from build123d import *

# Parameters (mm, degrees)
F1_DEPTH = 500
F2_W     = 221.745663
F2_H     = 538.323703
F2_R     = 1.9
F3_DEPTH = 50
F4_W     = 4.4
F4_H     = 51
F4_W_2   = 12.8
F4_R     = 1.9
F5_DEPTH = 1


with BuildPart() as f1:
    # F0 (on Front) → F1 (new body)
    with BuildSketch(Plane.XZ):
        with BuildLine():
            Line((-20, 3), (-20, 42))
            Line((-20, 42), (-23, 42))
            Line((-23, 42), (-23, 3))
            ThreePointArc((-23, 3), (-21.242641, -1.242641), (-17, -3))
            Line((-17, -3), (127, -3))
            Line((127, -3), (127, 0))
            Line((127, 0), (-17, 0))
            ThreePointArc((-17, 0), (-19.12132, 0.87868), (-20, 3))
        make_face()
    extrude(amount=-F1_DEPTH)

    # F2 (on Top) → F3 (cut, symmetric)
    with BuildSketch(Plane.XY):
        with Locations((54.499505, 256.060087)):
            Rectangle(F2_W, F2_H)
        with BuildLine():
            Line((126.619398, 279.652744), (33.186834, 54.086583))
            ThreePointArc((33.186834, 54.086583), (31.345288, 51.842652), (28.567437, 51))
            Line((28.567437, 51), (-3.3, 51))
            ThreePointArc((-3.3, 51), (-5.421321, 50.12132), (-6.3, 48))
            Line((-6.3, 48), (-6.3, 0))
            Line((-6.3, 0), (-16, 0))
            Line((-16, 0), (-16, 16))
            ThreePointArc((-16, 16), (-16.87868, 18.12132), (-19, 19))
            Line((-19, 19), (-23, 19))
            Line((-23, 19), (-23, 397))
            ThreePointArc((-23, 397), (-20.832031, 401.120631), (-16.20816, 401.667902))
            Line((-16.20816, 401.667902), (123.79184, 347.926937))
            ThreePointArc((123.79184, 347.926937), (126.120631, 346.091066), (127, 343.259035))
            Line((127, 343.259035), (127, 281.566161))
            ThreePointArc((127, 281.566161), (126.903926, 280.59071), (126.619398, 279.652744))
        make_face(mode=Mode.SUBTRACT)
        Polygon((467.411696, 344.689719), (455.614504, 344.432303), (456.010659, 326.276753), (456.727063, 293.44444), (469.524017, 293.72367), (468.411458, 344.711534), align=None)
        with Locations((461.573169, 300.551848)):
            Circle(F2_R, mode=Mode.SUBTRACT)
        with Locations((461.169593, 319.047446)):
            Circle(F2_R, mode=Mode.SUBTRACT)
        with Locations((460.766018, 337.543043)):
            Circle(F2_R, mode=Mode.SUBTRACT)
        Polygon((472.810411, 344.807519), (468.411458, 344.711534), (469.524017, 293.72367), (473.92297, 293.819656), align=None)
        Polygon((485.607364, 345.08675), (472.810411, 344.807519), (473.92297, 293.819656), (474.922732, 293.841471), (486.719924, 294.098886), align=None)
        with Locations((481.568409, 300.988146)):
            Circle(F2_R, mode=Mode.SUBTRACT)
        with Locations((481.164834, 319.483744)):
            Circle(F2_R, mode=Mode.SUBTRACT)
        with Locations((480.761259, 337.979341)):
            Circle(F2_R, mode=Mode.SUBTRACT)
        with Locations((-11.3, 44)):
            Circle(F2_R)
        with Locations((-11.3, 25.5)):
            Circle(F2_R)
        with Locations((-11.3, 7)):
            Circle(F2_R)
    extrude(amount=F3_DEPTH, both=True, mode=Mode.SUBTRACT)

    # F4 (on face) → F5 (join)
    with BuildSketch(Plane(origin=(0, 0, -3), x_dir=(1, 0, 0), z_dir=(0, 0, -1))):
        with Locations((-21.3, -25.5)):
            Rectangle(F4_W, F4_H)
        with Locations((-12.7, -25.5)):
            Rectangle(F4_W_2, F4_H)
        with Locations((-11.3, -44)):
            Circle(F4_R, mode=Mode.SUBTRACT)
        with Locations((-11.3, -25.5)):
            Circle(F4_R, mode=Mode.SUBTRACT)
        with Locations((-11.3, -7)):
            Circle(F4_R, mode=Mode.SUBTRACT)
    extrude(amount=F5_DEPTH)


solid = f1.part
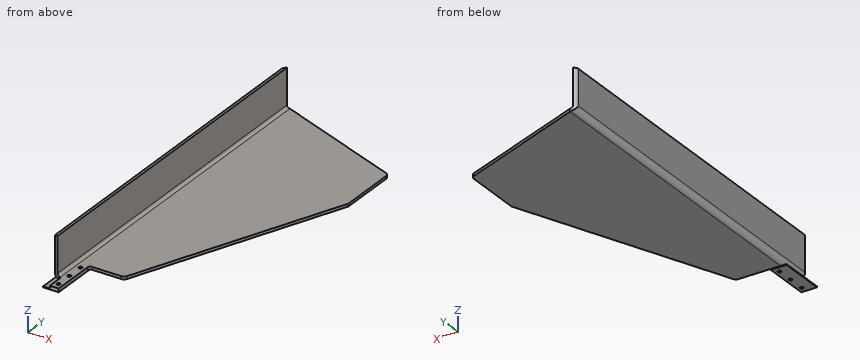
CAD build for the part. Positions are in the model's coordinates, mm. Give positions to 0.01 mm unless a question says otherwise; leave off trailing zeros. Write each loop counter-clockwise with the first axis right and the second up, starting at its lowest first coordinate (ties: lowest second). Pieces come first, ordered by that corner, then holes. Notation, with made-up numbers: (10, -12.5) - (28, -12.5) arc R26 ccw to (28, 6.5) - close; hole circle Ø4 at (70, 48). An arc over 180 degrees is marked (long way). Answer as CSV lines item,"result".
Q1. Band-saw the part on A-A (y = 336). Give the cut face in (x, z).
Result set:
outline,"(-23, 3) arc R6 ccw to (-17, -3) - (127, -3) - (127, 0) - (-17, 0) arc R3 cw to (-20, 3) - (-20, 42) - (-23, 42) - close"
Q2. Flat gauge pins, fed straight in: pin 1 Ø3.5 at (y, z) = (11, -1.5) entering from -X; pin 2 Ø1 at (x, y) = (10.5, 351.5) entering from -Z; pin 3 Ø1 at (y, z) = (301.5, 8.5) entering from -X; pin 4 Ø2.5 at (x, z) = (12.5, -1) entering from -Y. Where does each tip first touch, or does it go through?
Result set:
pin 1,"x = -23.5"
pin 2,"z = -3"
pin 3,"x = -23"
pin 4,"y = 51"
Q3. Drill centre lines: line 1 (Y direction, x = -11.3, z = -3.6); line 2 (Y direction, x = -11, z = -1); line 3 (Z direction, x = 80, y = 232.5). Where is each one in solid material? Low to high. Write a range as from..to.
Result set:
line 1,"0..5.1, 8.9..23.6, 27.4..42.1, 45.9..51"
line 2,"0..5.12, 8.88..23.62, 27.38..42.12, 45.88..399.67"
line 3,"-3..0"
Q4. Band-saw the part on D-D (y = 87). Give the cut face in (x, z).
Result set:
outline,"(-23, 3) arc R6 ccw to (-17, -3) - (46.82, -3) - (46.82, 0) - (-17, 0) arc R3 cw to (-20, 3) - (-20, 42) - (-23, 42) - close"
Q5. Band-saw the part on C-C (x = 40). Give the cut face in (y, z), and give its area (3 significant figures).
Result set:
outline,"(70.54, -3) - (380.09, -3) - (380.09, 0) - (70.54, 0) - close"
area,"929 mm²"
Q6. Band-saw the part on B-B (z = 28). Give the cut face in (x, y).
Result set:
outline,"(-23, 19) - (-20, 19) - (-20, 401.58) arc R5 ccw to (-23, 397) - close"
